from build123d import *

# Parameters (mm, degrees)
SKETCH_1_W          = 600
SKETCH_1_H          = 200
EXTRUDE_1_DEPTH     = 10
SKETCH_2_R          = 2
EXTRUDE_2_DEPTH     = 100
SKETCH_3_W          = 100
SKETCH_3_H          = 200
SKETCH_3_W_2        = 50
CUT_EXTRUDE_1_DEPTH = 10


with BuildPart() as part:
    # 草图1 → 凸台-拉伸1 (new body)
    with BuildSketch(Plane(origin=(0, 0, 0), x_dir=(1, 0, 0), z_dir=(0, 1, 0))):
        Rectangle(SKETCH_1_W, SKETCH_1_H)
    extrude(amount=-EXTRUDE_1_DEPTH)

    # 草图2 → 凸台-拉伸2 (add)
    with BuildSketch(Plane(origin=(0, 0, 0), x_dir=(1, 0, 0), z_dir=(0, 1, 0))):
        with Locations(Location((-129.5, 39, 0), (0, 0, 90))):
            Circle(SKETCH_2_R)
        with Locations(Location((-129.5, -39, 0), (0, 0, 90))):
            Circle(SKETCH_2_R)
        with Locations(Location((74.5, 25, 0), (0, 0, 90))):
            Circle(SKETCH_2_R)
        with Locations(Location((74.5, -25, 0), (0, 0, 90))):
            Circle(SKETCH_2_R)
    extrude(amount=EXTRUDE_2_DEPTH)

    # 草图3 → 切除-拉伸1 (cut)
    with BuildSketch(Plane(origin=(0, 0, 0), x_dir=(1, 0, 0), z_dir=(0, 1, 0))):
        with Locations((-250, 0)):
            Rectangle(SKETCH_3_W, SKETCH_3_H)
        with Locations((275, 0)):
            Rectangle(SKETCH_3_W_2, SKETCH_3_H)
    extrude(amount=-CUT_EXTRUDE_1_DEPTH, mode=Mode.SUBTRACT)


solid = part.part
The model under review builds one solid part; all positions refer to its coordinate system, in mm. Round coordinates to 2 decimals unless told otherwise and drop trailing zeros. Order: outer loops, then holes, each group sorted by start corner. A loop starts at its lowest first (then second) coordinate and runs counter-clockwise, first axis right, second up. Notation, with made-up numbers: (24, 2.25) -> (60, 2.25) arc R27 cw to (60, 29.25) -> close; hole circle Ø11 at (1, 15). An arc over 180 degrees is marked (long way). Return JSON: item names as keys, results as strings.
1. Insertion check: P1, Ø5, axis at x = 78.5, y = 78.5, coming from the -Z side. The pin has a flat end and moves straight along its axis. Give the tip position at first contact, or say it passes through.
Answer block:
{"P1": "stops at z = -26.32"}
2. For L1, parallel to Y at x = 60, z = 48; L2, parallel to X at y = 75.5, z = -25, list the stretches that pass through material, from the lowest coordinate up. Write a range as [from, to].
Answer block:
{"L1": "y = [-10, 0]", "L2": "x = [72.5, 76.5]"}
3. Take a section at B-B (x = -18.5). Write out the cut boundary in (y, z).
Answer block:
{"outline": "(-10, -100) -> (0, -100) -> (0, 100) -> (-10, 100) -> close"}
4. Take a section at C-C (z = -31.5). Write out the cut boundary in (x, y), then the cut area to 3 significant figures.
Answer block:
{"outline": "(-200, -10) -> (250, -10) -> (250, 0) -> (-200, 0) -> close", "area": "4,500 mm²"}
5. Take a section at A-A (y = 16.5). Write out the cut boundary in (x, z), then the cut area to 3 significant figures.
Answer block:
{"outline": "circle Ø4 at (-129.5, -39); circle Ø4 at (-129.5, 39); circle Ø4 at (74.5, -25); circle Ø4 at (74.5, 25)", "area": "50.3 mm²"}
